from build123d import *

# Parameters (mm, degrees)
REVOLVE1_ANGLE      = 180
SKETCH4_R           = 11.5
BOSS_EXTRUDE1_DEPTH = 20
SKETCH5_R           = 1.55
CUT_EXTRUDE1_DEPTH  = 11.5


with BuildPart() as part:
    # Sketch1 → Revolve1 (revolve)
    with BuildSketch(Plane(origin=(0, 0, 0), x_dir=(1, 0, 0), z_dir=(0, 1, 0))):
        with BuildLine():
            Line((0, 11.5), (0, -11.5))
            ThreePointArc((0, -11.5), (-11.5, 0), (0, 11.5))
        make_face()
    revolve(axis=Axis((0, 0, -22.021429017), (0, 0, 1)), revolution_arc=REVOLVE1_ANGLE)

    # Sketch4 → Boss-Extrude1 (add)
    with BuildSketch(Plane(origin=(0, 0, 0), x_dir=(1, 0, 0), z_dir=(0, 1, 0))):
        with Locations(Location((0, 0, 0), (0, 0, 180))):
            Circle(SKETCH4_R)
    extrude(amount=BOSS_EXTRUDE1_DEPTH)

    # Sketch5 → Cut-Extrude1 (cut, symmetric)
    with BuildSketch(Plane.XY):
        with Locations((0, 10)):
            Circle(SKETCH5_R)
    extrude(amount=CUT_EXTRUDE1_DEPTH, both=True, mode=Mode.SUBTRACT)


solid = part.part
The listing builds one solid part. Answer for the finished solid, in the listing's coordinates (mm). Coordinates: 2 decimals unless noted, no trailing zeros. Loops run counter-clockwise (first coordinate to the right, second up) from the corner with the lowest first, then second, coordinate; pieces in that order, holes last.
1) Find section C-C on y = 10. Write down the section's boundary in (x, z).
2) Find section A-A on x = 0. Write down the section's boundary in (y, z), then the cut area to 3 significant figures.
3) Flat-ended cylindrical pins translate along their axes: pin 1 Ø6 at (x, y) = (-8.5, 3) entering from -Z; pin 2 Ø1.5 at (x, y) = (-0.5, -8.5) entering from -Z; pin 3 Ø3 at (y, z) = (3.5, 6) entering from -X. Find the tip coordinate at first contact, or state that the pin passes through.
4) Determine the mould class of faces 1 (the face through (2.493, 9.86, -11.227)), 2 (the face through (0, 20, 0)), 3 (the face through (0.715, 8.625, 0.161)) for opening direction X: pulls with the +X half, pulls with the -X half, needs draft (parallel to the pull), parting line crosses it, or undercut.
5) Find the intervals of material crossed by L1, parallel to Y at x = 0, z = 0; L2, parallel to X at y = 10, z = 3.5; L3, parallel to Y at x = 0, z = 4.75, in increasing order.
6) Find section D-D on y = 0.5. Write down the section's boundary in (x, z).
7) Find section B-B on z = 0. Write down the section's boundary in (x, y).
Values:
1. outline: (-1.55, -11.4) - (-1.55, 11.4) arc R11.5 ccw to start; (1.55, -11.4) arc R11.5 ccw to (1.55, 11.4) - close
2. outline: (0, -11.5) - (8.45, -11.5) - (8.45, 11.5) - (0, 11.5) arc R11.5 ccw to start; (11.55, -11.5) - (20, -11.5) - (20, 11.5) - (11.55, 11.5) - close
2. area: 596 mm2
3. pin 1: stops at z = -10.1
3. pin 2: stops at z = -8.48
3. pin 3: stops at x = -10.58
4. face 1: parting line crosses it
4. face 2: needs draft
4. face 3: undercut
5. L1: y = -11.5 to 8.45, 11.55 to 20
5. L2: x = -10.95 to -1.55, 1.55 to 10.95
5. L3: y = -10.47 to 8.45, 11.55 to 20
6. outline: circle Ø23 at (0, 0)
7. outline: (-11.5, 0) arc R11.5 ccw to (11.5, 0) - (11.5, 20) - (-11.5, 20) - close; hole circle Ø3.1 at (0, 10)
